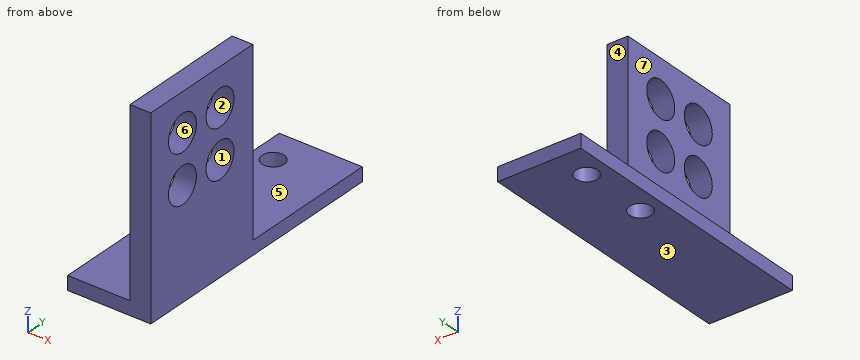
```python
from build123d import *

# Parameters (mm, degrees)
FOOT_SKETCH_W              = 12
FOOT_SKETCH_H              = 39.4
FOOT_DEPTH                 = 2
UPRIGHT_SKETCH_W           = 3
UPRIGHT_SKETCH_H           = 19
UPRIGHT_DEPTH              = 26.2
SHEATH_HOLES_SKETCH_R      = 2.6
SHEATH_HOLES_DEPTH         = 3
SERVO_SCREW_HOLES_SKETCH_R = 1.6
SERVO_SCREW_HOLES_DEPTH    = 15


with BuildPart() as part:
    # Foot Sketch → Foot (new body)
    with BuildSketch(Plane.XY.offset(-4)):
        with Locations((-73.35, 73.7)):
            Rectangle(FOOT_SKETCH_W, FOOT_SKETCH_H)
    extrude(amount=FOOT_DEPTH)

    # Upright Sketch → Upright (add)
    with BuildSketch(Plane.XY.offset(-2)):
        with Locations((-68.85, 63.5)):
            Rectangle(UPRIGHT_SKETCH_W, UPRIGHT_SKETCH_H)
    extrude(amount=UPRIGHT_DEPTH)

    # Sheath Holes Sketch → Sheath Holes (cut)
    with BuildSketch(Plane(origin=(-70.35, 0, 0), x_dir=(0, 0, -1), z_dir=(1, 0, 0))):
        with Locations((-18.7, 66.9)):
            Circle(SHEATH_HOLES_SKETCH_R)
        with Locations((-11.7, 59.9)):
            Circle(SHEATH_HOLES_SKETCH_R)
        with Locations((-11.7, 66.9)):
            Circle(SHEATH_HOLES_SKETCH_R)
        with Locations((-18.7, 59.9)):
            Circle(SHEATH_HOLES_SKETCH_R)
    extrude(amount=SHEATH_HOLES_DEPTH, mode=Mode.SUBTRACT)

    # Servo Screw Holes Sketch → Servo Screw Holes (cut, symmetric)
    with BuildSketch(Plane.XY):
        with Locations((-76.35, 78.4)):
            Circle(SERVO_SCREW_HOLES_SKETCH_R)
        with Locations((-76.35, 88.4)):
            Circle(SERVO_SCREW_HOLES_SKETCH_R)
    extrude(amount=SERVO_SCREW_HOLES_DEPTH, both=True, mode=Mode.SUBTRACT)


solid = part.part
```
The listing builds one solid part. Answer for the finished solid, in the listing's coordinates (mm). Face numbers are marked on the shaded views. A direction names the side the tool comes from. Give positions to 0.01 mm unless a question says otherwise; leave off trailing zeros. Loops run counter-clockwise (first coordinate to the right, second up) from the corner with the lowest first, then second, coordinate; pieces in that order, holes last. Notation, with made-up numbers: (31.25, 33) - (74.25, 33) arc R14 ccw to (74.25, 44) - close; hole circle Ø10 at (2.5, 15). An arc over 180 degrees is marked (long way). Return JSON: item names as keys, results as strings. Group by question number.
1. Determine the mould class of the marked faces 1, 2, 3 and 4 for opening direction Z: pulls with the +Z half, pulls with the -Z half, needs draft (parallel to the pull), parting line crosses it, or undercut.
2. Which of the six approach directions +Z, -Z, +X, -X, +Y, -Y give full straight-line access (tool end or side, diameter ignored) to the marked faces 5, 6 and 7?
3. Find section A-A (x = -76.35). Write down the section's boundary in (y, z), then the cut area to 3 significant figures.
4. Given pin 1 Ø8.5 at (y, z) = (66.9, 11.7) entering from +X; pin 2 Ø4 at (x, y) = (-74, 66) entering from +Z; pin 3 Ø8.5 at (y, z) = (59.9, 11.7) entering from -X; pin 4 Ø1.5 at (x, z) = (-69.5, 15.5) entering from +Y, each flat-ended and moving along its own axis, determine where each tip first touches the part or whether it passes through.
5. Find section D-D (x = -69.25). Write down the section's boundary in (y, z), then the cut area to 3 significant figures.
6. Find section C-C (y = 88.4). Write down the section's boundary in (x, z), then the cut area to 3 significant figures.
7. Find section B-B (z = 11.7). Write down the section's boundary in (x, y).
8. Straight lines are drawn through the part: line 1 (Y direction, x = -69.5, z = 11.7); line 2 (Y direction, x = -76.35, z = -3.15); line 3 (Z direction, x = -69, y = 59). For each, find the intervals that lie inside material, in ascending order. Write a range as [from, to].
Verdict:
{
 "1": {"face 1": "undercut", "face 2": "undercut", "face 3": "pulls with the -Z half", "face 4": "needs draft"},
 "2": {"face 5": "+Z, -X, +Y", "face 6": "+X, -X", "face 7": "+Z, -X, +Y, -Y"},
 "3": {"outline": "(54, -4) - (76.8, -4) - (76.8, -2) - (54, -2) - close; (80, -4) - (86.8, -4) - (86.8, -2) - (80, -2) - close; (90, -4) - (93.4, -4) - (93.4, -2) - (90, -2) - close", "area": "66.0 mm^2"},
 "4": {"pin 1": "stops at x = -67.35", "pin 2": "stops at z = -2", "pin 3": "stops at x = -70.35", "pin 4": "stops at y = 73"},
 "5": {"outline": "(54, -4) - (93.4, -4) - (93.4, -2) - (73, -2) - (73, 24.2) - (54, 24.2) - close; hole circle Ø5.2 at (59.9, 11.7); hole circle Ø5.2 at (59.9, 18.7); hole circle Ø5.2 at (66.9, 11.7); hole circle Ø5.2 at (66.9, 18.7)", "area": "492 mm^2"},
 "6": {"outline": "(-79.35, -4) - (-77.95, -4) - (-77.95, -2) - (-79.35, -2) - close; (-74.75, -4) - (-67.35, -4) - (-67.35, -2) - (-74.75, -2) - close", "area": "17.6 mm^2"},
 "7": {"outline": "(-70.35, 54) - (-67.35, 54) - (-67.35, 57.3) - (-70.35, 57.3) - close; (-70.35, 62.5) - (-67.35, 62.5) - (-67.35, 64.3) - (-70.35, 64.3) - close; (-70.35, 69.5) - (-67.35, 69.5) - (-67.35, 73) - (-70.35, 73) - close"},
 "8": {"line 1": "y = [54, 57.3], [62.5, 64.3], [69.5, 73]", "line 2": "y = [54, 76.8], [80, 86.8], [90, 93.4]", "line 3": "z = [-4, 9.26], [14.14, 16.26], [21.14, 24.2]"}
}
